from build123d import *

# Parameters (mm, degrees)
DODANIE_WYCI_GNI_CIE1_DEPTH = 5
OTW_R_POD_RUB_M21_D         = 2.6
OTW_R_POD_RUB_M21_DEPTH     = 5
OTW_R_POD_RUB_M51_D         = 5.8
OTW_R_POD_RUB_M51_DEPTH     = 5
OTW_R_POD_RUB_M22_D         = 2.6
OTW_R_POD_RUB_M22_DEPTH     = 5


with BuildPart() as part:
    # Szkic1 → Dodanie-wyciągnięcie1 (new body)
    with BuildSketch(Plane.XY):
        with BuildLine():
            Line((-25, 4), (25, 4))
            ThreePointArc((25, 4), (26.414213562, 3.414213562), (27, 2))
            Line((27, 2), (27, -2))
            ThreePointArc((27, -2), (26.414213562, -3.414213562), (25, -4))
            Line((25, -4), (-25, -4))
            ThreePointArc((-25, -4), (-26.414213562, -3.414213562), (-27, -2))
            Line((-27, -2), (-27, 2))
            ThreePointArc((-27, 2), (-26.414213562, 3.414213562), (-25, 4))
        make_face()
    extrude(amount=DODANIE_WYCI_GNI_CIE1_DEPTH)

    # Otwór pod śrubę M21
    with Locations(Plane.XY.offset(5)):
        with Locations((-10, 0), (21.75, 0)):
            Hole(OTW_R_POD_RUB_M21_D / 2, depth=OTW_R_POD_RUB_M21_DEPTH)

    # Otwór pod śrubę M51
    with Locations(Plane.XY.offset(5)):
        with Locations((6, 0)):
            Hole(OTW_R_POD_RUB_M51_D / 2, depth=OTW_R_POD_RUB_M51_DEPTH)

    # Otwór pod śrubę M22
    with Locations(Plane.XY.offset(5)):
        with Locations((-24, 0)):
            Hole(OTW_R_POD_RUB_M22_D / 2, depth=OTW_R_POD_RUB_M22_DEPTH)


solid = part.part
Can you work these out from the model? Positions are in its coordinate system, mm. Coordinates: 2 decimals unless noted, no trailing zeros. Loops run counter-clockwise (first coordinate to the right, second up) from the corner with the lowest first, then second, coordinate; pieces in that order, holes last. Notation, with made-up numbers: M 71.5,37.5 L 130.5,37.5 A15 cw 130.5,43.5 Z; hole C 82,85 d2. An arc over 180 degrees is marked long. Return JSON: item names as keys, results as strings. Group by question number.
Item 1: Imagine slicing it at D-D (x = 6). Please give me the cut outline in (y, z).
Item 2: If I drill on L1, parallel to Y at x = 6, z = 1.45; L2, parallel to Y at x = 21.75, z = 1; L3, parallel to X at y = 0.5, z = 0.9, over which ranges is the centre line in solid material (lowest first)? Write a range as from..to.
Item 3: Thinking about a two-plate mould opening in X: for faces 1 (the cylindrical face through (26.43, -3.4, 2.46)), 2 (the cylindrical face through (-11.24, 0.39, 2.46)), 3 (the flat face through (0, 0, 5)), which applies, released by +X, released by -X, zero draft, split by the parting line, or undercut?
Item 4: I'm going to push a flat-ended pin straight in: pin 1 Ø3.5 at (x, y) = (-10, 0) entering from -Z. Where does the tip first touch, or does it pass through?
Item 5: Imagine slicing it at A-A (z = 1.5). Please give me the cut outline in (x, y), and give its area (3 significant figures).
Item 6: Imagine slicing it at B-B (x = -10). Please give me the cut outline in (y, z), and give its area (3 significant figures).
Item 7: Imagine slicing it at C-C (y = 0). Please give me the cut outline in (x, z).
Verdict:
{
 "1": {"outline": "M -4,0 L -2.9,0 L -2.9,5 L -4,5 Z; M 2.9,0 L 4,0 L 4,5 L 2.9,5 Z"},
 "2": {"L1": "y = -4..-2.9, 2.9..4", "L2": "y = -4..-1.3, 1.3..4", "L3": "x = -27..-25.2, -22.8..-11.2, -8.8..3.14, 8.86..20.55, 22.95..27"},
 "3": {"face 1": "released by +X", "face 2": "undercut", "face 3": "zero draft"},
 "4": {"pin 1": "stops at z = 0"},
 "5": {"outline": "M -27,-2 A2 ccw -25,-4 L 25,-4 A2 ccw 27,-2 L 27,2 A2 ccw 25,4 L -25,4 A2 ccw -27,2 Z; hole C -24,0 d2.6; hole C -10,0 d2.6; hole C 6,0 d5.8; hole C 21.75,0 d2.6", "area": "386 mm^2"},
 "6": {"outline": "M -4,0 L -1.3,0 L -1.3,5 L -4,5 Z; M 1.3,0 L 4,0 L 4,5 L 1.3,5 Z", "area": "27.0 mm^2"},
 "7": {"outline": "M -27,0 L -25.3,0 L -25.3,5 L -27,5 Z; M -22.7,0 L -11.3,0 L -11.3,5 L -22.7,5 Z; M -8.7,0 L 3.1,0 L 3.1,5 L -8.7,5 Z; M 8.9,0 L 20.45,0 L 20.45,5 L 8.9,5 Z; M 23.05,0 L 27,0 L 27,5 L 23.05,5 Z"}
}
